```python
from build123d import *

# Parameters (mm, degrees)
SKETCH2_W           = 38.1
SKETCH2_H           = 69.85
SKETCH2_R           = 1.4732
SKETCH2_W_2         = 27.6098
SKETCH2_H_2         = 57.15
BOSS_EXTRUDE1_DEPTH = 6.0452


with BuildPart() as part:
    # Sketch2 → Boss-Extrude1 (new body)
    with BuildSketch(Plane(origin=(0, 0, 0), x_dir=(1, 0, 0), z_dir=(0, 1, 0))):
        with Locations((-7.173243467, 10.249774524)):
            Rectangle(SKETCH2_W, SKETCH2_H)
        with Locations(Location((-7.173243467, 41.999774524, 0), (0, 0, 90))):
            Circle(SKETCH2_R, mode=Mode.SUBTRACT)
        with Locations(Location((-7.173243467, -21.500225476, 0), (0, 0, 270))):
            Circle(SKETCH2_R, mode=Mode.SUBTRACT)
        with Locations((-7.173243467, 10.249774524)):
            Rectangle(SKETCH2_W_2, SKETCH2_H_2, mode=Mode.SUBTRACT)
    extrude(amount=BOSS_EXTRUDE1_DEPTH)


solid = part.part
```
Can you work these out from the model? Positions are in its coordinate system, mm. A direction names the side the tool comes from. Coordinates: 2 decimals unless noted, no trailing zeros. Order: outer loops, then holes, each group sorted by start corner. A loop starts at its lowest first (then second) coordinate and runs counter-clockwise, first axis right, second up.
1. I'm going to push a flat-ended pin straight in: pin 1 (4.5 mm diameter, centred on x = -7.17, z = 21.5, fed in from -Y). Where does the tip first touch, or does it pass through?
2. I need wall thicknesses on line 1 (X direction, y = 3.75, z = -11); line 2 (Z direction, x = -18, y = 4); line 3 (Z direction, x = -8.5, y = 2.5). Which ranges of each line are inside material? Lowest first, please.
3. For faces 5 (the face through (-20.978, 3, -10)), 6 (the face through (11.877, 3, -10)), which set-ups out of +Z, -Z, +X, -X, +Y, -Y let a thin tool reach every point of the face, with its end or its side?
4. Thinking about a two-plate mould opening in X: for faces 1 (the face through (-7.11, 2.98, 20.03)), 2 (the face through (-7, 3, -45.175)), 3 (the face through (6.632, 3, -10)), 4 (the face through (-26.223, 3, -10)), which applies, +X half, -X half, draft (parallel to the pull), parting line (faces both ways), or undercut?
5. If we section it at C-C (y = 5): Please give me the cut outline in (x, z), then the cut area to 3 significant figures.
6. If we section it at B-B (x = -18.5): Please give me the cut outline in (y, z), then the cut area to 3 significant figures.
7. If we section it at A-A (z = -8): Please give me the cut outline in (x, y), then the cut area to 3 significant figures.
Entries:
1. pin 1: stops at y = 0
2. line 1: x = -26.22 to -20.98, 6.63 to 11.88
2. line 2: z = -45.17 to -38.82, 18.33 to 24.68
2. line 3: z = -45.17 to -42.64, -41.36 to -38.82, 18.33 to 20.86, 22.14 to 24.68
3. face 5: +Y, -Y
3. face 6: +Z, -Z, +X, +Y, -Y
4. face 1: undercut
4. face 2: draft
4. face 3: undercut
4. face 4: -X half
5. outline: (-26.22, -45.17) - (11.88, -45.17) - (11.88, 24.68) - (-26.22, 24.68) - close; hole (-20.98, -38.82) - (6.63, -38.82) - (6.63, 18.33) - (-20.98, 18.33) - close; hole circle Ø2.95 at (-7.17, -42); hole circle Ø2.95 at (-7.17, 21.5)
5. area: 1,070 mm2
6. outline: (0, -45.17) - (6.05, -45.17) - (6.05, -38.82) - (0, -38.82) - close; (0, 18.33) - (6.05, 18.33) - (6.05, 24.68) - (0, 24.68) - close
6. area: 76.8 mm2
7. outline: (-26.22, 0) - (-20.98, 0) - (-20.98, 6.05) - (-26.22, 6.05) - close; (6.63, 0) - (11.88, 0) - (11.88, 6.05) - (6.63, 6.05) - close
7. area: 63.4 mm2
